from build123d import *

# Parameters (mm, degrees)
CROQUIS1_R              = 2.5
CROQUIS1_R_2            = 2.821368504
SALIENTE_EXTRUIR1_DEPTH = 4


with BuildPart() as part:
    # Croquis1 → Saliente-Extruir1 (new body)
    with BuildSketch(Plane.XY):
        with BuildLine():
            Line((26.393375205, 6.699416954), (97.693375205, 6.699416954))
            ThreePointArc((97.693375205, 6.699416954), (102.183503265, 4.839545014), (104.043375205, 0.349416954))
            Line((104.043375205, 0.349416954), (104.043375205, -0.895643676))
            ThreePointArc((104.043375205, -0.895643676), (105.507841299, -4.431177582), (109.043375205, -5.895643676))
            Line((109.043375205, -5.895643676), (119.043375205, -5.895643676))
            ThreePointArc((119.043375205, -5.895643676), (122.578909111, -4.431177582), (124.043375205, -0.895643676))
            Line((124.043375205, -0.895643676), (124.043375205, 6.604356324))
            Line((124.043375205, 6.604356324), (124.043375205, 20.254356324))
            ThreePointArc((124.043375205, 20.254356324), (122.183503265, 24.744484385), (117.693375205, 26.604356324))
            Line((117.693375205, 26.604356324), (6.393375205, 26.604356324))
            ThreePointArc((6.393375205, 26.604356324), (1.903247144, 24.744484385), (0.043375205, 20.254356324))
            Line((0.043375205, 20.254356324), (0.043375205, 6.604356324))
            Line((0.043375205, 6.604356324), (0.043375205, -17.045643676))
            ThreePointArc((0.043375205, -17.045643676), (1.903247144, -21.535771736), (6.393375205, -23.395643676))
            Line((6.393375205, -23.395643676), (13.693375205, -23.395643676))
            ThreePointArc((13.693375205, -23.395643676), (18.183503265, -21.535771736), (20.043375205, -17.045643676))
            Line((20.043375205, -17.045643676), (20.043375205, 0.349416954))
            ThreePointArc((20.043375205, 0.349416954), (21.903247144, 4.839545014), (26.393375205, 6.699416954))
        make_face()
        with Locations((10.043375205, 15.866498333)):
            Circle(CROQUIS1_R, mode=Mode.SUBTRACT)
        with Locations((114.183375205, 15.771437703)):
            Circle(CROQUIS1_R_2, mode=Mode.SUBTRACT)
        with Locations((10.043375205, -6.395643676)):
            Circle(CROQUIS1_R, mode=Mode.SUBTRACT)
        with Locations((62.043375205, 15.866498333)):
            Circle(CROQUIS1_R_2, mode=Mode.SUBTRACT)
        with Locations((114.183375205, 0.104356324)):
            Circle(CROQUIS1_R_2, mode=Mode.SUBTRACT)
    extrude(amount=SALIENTE_EXTRUIR1_DEPTH)


solid = part.part
Can you work these out from the model? Positions are in its coordinate system, mm. A direction names the side the tool comes from. Give positions to 0.01 mm unless a question says otherwise; leave off trailing zeros. Loops run counter-clockwise (first coordinate to the right, second up) from the corner with the lowest first, then second, coordinate; pieces in that order, holes last. Notation, with made-up numbers: (61, -40) - (115, -40) arc R31 cw to (115, -9) - close; hole circle Ø2 at (52.5, 72.25). An arc over 180 degrees is marked (long way). Answer as a JSON object with one key per item and string values.
Q1. Imagine slicing it at A-A on x = 60.5. Write out the boundary of the cut face in (y, z), plus the area to 3 significant figures.
Geometry says:
{"outline": "(6.7, 0) - (13.5, 0) - (13.5, 4) - (6.7, 4) - close; (18.23, 0) - (26.6, 0) - (26.6, 4) - (18.23, 4) - close", "area": "60.7 mm²"}
Q2. Imagine slicing it at B-B on z = 2.4. Write out the boundary of the cut face in (x, y).
Geometry says:
{"outline": "(0.04, -17.05) arc R6.35 ccw to (6.39, -23.4) - (13.69, -23.4) arc R6.35 ccw to (20.04, -17.05) - (20.04, 0.35) arc R6.35 cw to (26.39, 6.7) - (97.69, 6.7) arc R6.35 cw to (104.04, 0.35) - (104.04, -0.9) arc R5 ccw to (109.04, -5.9) - (119.04, -5.9) arc R5 ccw to (124.04, -0.9) - (124.04, 20.25) arc R6.35 ccw to (117.69, 26.6) - (6.39, 26.6) arc R6.35 ccw to (0.04, 20.25) - close; hole circle Ø5 at (10.04, -6.4); hole circle Ø5 at (10.04, 15.87); hole circle Ø5.64 at (62.04, 15.87); hole circle Ø5.64 at (114.18, 0.1); hole circle Ø5.64 at (114.18, 15.77)"}
Q3. If I drill on L1, parallel to X at y = 16, z = 1.45; L2, parallel to X at y = 0, z = 2.9; L3, parallel to X at y = -1.5, z = 0.8, over which ranges is the centre line in solid material (lowest first)?
Geometry says:
{"L1": "0.04 to 7.55, 12.54 to 59.23, 64.86 to 111.37, 117 to 124.04", "L2": "0.04 to 20.04, 104.04 to 111.36, 117 to 124.04", "L3": "0.04 to 20.04, 104.08 to 111.86, 116.5 to 124.01"}
Q4. If we mould it in two halves opening along X, with no side actions, what happens to faces 1 (the cylindrical face through (122.54, -4.47, 1.97)), 2 (the cylindrical face through (21.854, 4.79, 1.972)), 3 (the cylindrical face through (1.854, -21.486, 1.972))? For each: pulls with the +X half, pulls with the -X half, needs draft (parallel to the pull), parting line crosses it, or undercut.
Geometry says:
{"face 1": "pulls with the +X half", "face 2": "undercut", "face 3": "pulls with the -X half"}
Q5. Will these pins go through, and if not, where does the flat tip stop? P1, Ø1.2, axis at x = 79, z = 2, coming from the -Y side; P2, Ø8, axis at x = 10.04, y = -6.4, coming from the -Z side; P3, Ø2, axis at x = 116.5, z = 1, coming from the -Y side.
Geometry says:
{"P1": "y = 6.7", "P2": "z = 0", "P3": "y = -5.9"}
Q6. Which directions (+Z, -Z, +X, -X, +Y, -Y) give clear straight access to the entire face, cutting with the end or side of a thin tool? Please do faces 4 (the flat face through (114, -5.896, 2)), 5 (the flat face through (0.043, 2, 2)), 6 (the cylindrical face through (105.469, -4.392, 1.972)).
Geometry says:
{"face 4": "+Z, -Z, +X, -Y", "face 5": "+Z, -Z, -X, +Y, -Y", "face 6": "+Z, -Z, -Y"}
Q7. Imagine slicing it at D-D on x = 21.5. Write out the boundary of the cut face in (y, z), plus the area to 3 significant figures.
Geometry says:
{"outline": "(4.4, 0) - (26.6, 0) - (26.6, 4) - (4.4, 4) - close", "area": "88.8 mm²"}
Q8. Imagine slicing it at C-C on y = 5. Write out the boundary of the cut face in (x, z).
Geometry says:
{"outline": "(0.04, 0) - (22.07, 0) - (22.07, 4) - (0.04, 4) - close; (102.02, 0) - (124.04, 0) - (124.04, 4) - (102.02, 4) - close"}
